from build123d import *

# Parameters (mm, degrees)
BOX016_W     = 28
BOX016_H     = 4
BOX016_DEPTH = 10
BOX004_W     = 30
BOX004_H     = 8
BOX004_DEPTH = 2.5
BOX003_W     = 30
BOX003_H     = 10
BOX003_DEPTH = 3.5
BOX002_W     = 30
BOX002_H     = 21
BOX002_DEPTH = 1


with BuildPart() as cubo016:
    # Box016 → Box016 (new body)
    with BuildSketch(Plane(origin=(-13, -14, 0), x_dir=(1, 0, 0), z_dir=(0, 0, 1))):
        with Locations((14, 2)):
            Rectangle(BOX016_W, BOX016_H)
    extrude(amount=BOX016_DEPTH)


with BuildPart() as cubo004:
    # Box004 → Box004 (new body)
    with BuildSketch(Plane(origin=(-14, -15, 0), x_dir=(1, 0, 0), z_dir=(0, 0, 1))):
        with Locations((15, 4)):
            Rectangle(BOX004_W, BOX004_H)
    extrude(amount=BOX004_DEPTH)


with BuildPart() as cubo003:
    # Box003 → Box003 (new body)
    with BuildSketch(Plane(origin=(-14, -16, 0), x_dir=(1, 0, 0), z_dir=(0, 0, 1))):
        with Locations((15, 5)):
            Rectangle(BOX003_W, BOX003_H)
    extrude(amount=BOX003_DEPTH)


with BuildPart() as cut008:
    # Box002 → Box002 (new body)
    with BuildSketch(Plane(origin=(-14, -21, 0), x_dir=(1, 0, 0), z_dir=(0, 0, 1))):
        with Locations((15, 10.5)):
            Rectangle(BOX002_W, BOX002_H)
    extrude(amount=BOX002_DEPTH)

    # Fusion001: union Cubo003
    add(cubo003.part)

    # Cut006: cut Cubo004
    add(cubo004.part, mode=Mode.SUBTRACT)

    # Cut008: cut Cubo016
    add(cubo016.part, mode=Mode.SUBTRACT)


solid = cut008.part
Verification items for the finished model (mm, model axes). A direction names the side the tool comes from. Give positions to 0.01 mm unless a question says otherwise; leave off trailing zeros. Loops run counter-clockwise (first coordinate to the right, second up) from the corner with the lowest first, then second, coordinate; pieces in that order, holes last.
1. Material ranges on probe 1 along Y at (x, z) = (14, 2.65); probe 2 along Y at (x, z) = (11.5, 1.65); probe 3 along Z at (x, y) = (-10, -2), recorded low to high.
Derived:
probe 1: y = -16 to -14, -10 to -6
probe 2: y = -16 to -15, -7 to -6
probe 3: z = 0 to 1
2. Cross-section at A-A on x = -0.5. Record the cut outline in (y, z).
Derived:
outline: (-21, 0) - (-15, 0) - (-15, 2.5) - (-14, 2.5) - (-14, 3.5) - (-16, 3.5) - (-16, 1) - (-21, 1) - close; (-10, 2.5) - (-7, 2.5) - (-7, 0) - (0, 0) - (0, 1) - (-6, 1) - (-6, 3.5) - (-10, 3.5) - close
3. Tool access check on faces 1 (the flat face through (1, -7, 1)), 2 (the flat face through (1, -16, 2)), 3 (the flat face through (1, -3, 0)), 4 (the flat face through (1, -14, 3)), 5 (the flat face through (1, -3, 1)). Record the directions out of +Z, -Z, +X, -X, +Y, -Y that give a thin tool (end or side, any length) a straight path to the whole face; none if there is none.
Derived:
face 1: -Z, +X, -X
face 2: +Z, +X, -X, -Y
face 3: -Z, +X, -X, +Y, -Y
face 4: +Z, -Z
face 5: +Z, +X, -X, +Y
4. Release check for a two-part mould opening along X. For faces 6 (the flat face through (1, -18, 1)), 7 (the flat face through (-13, -12, 3)), 8 (the flat face through (16, -11, 3)) record: +X half, -X half, draft (parallel to the pull), parting line (faces both ways), or undercut.
Derived:
face 6: draft
face 7: undercut
face 8: +X half
5. Cross-section at C-C on y = -5.25. Record the cut outline in (x, z), and give its area (3 significant figures).
Derived:
outline: (-14, 0) - (16, 0) - (16, 1) - (-14, 1) - close
area: 30.0 mm2
6. Go/stop test with flat-tipped pins: P1, Ø6.5, axis at x = 6, y = -2, coming from the +Z side; P2, Ø1, axis at x = -6.5, z = 2.5, coming from the +Y side; P3, Ø0.5, axis at x = -2, z = 3, coming from the -Y side. Record where each tip stops, or that it passes through.
Derived:
P1: stops at z = 1
P2: stops at y = -6
P3: stops at y = -16
7. Cross-section at B-B on z = 1.5. Record the cut outline in (x, y), and give its area (3 significant figures).
Derived:
outline: (-14, -16) - (16, -16) - (16, -15) - (-14, -15) - close; (-14, -7) - (16, -7) - (16, -6) - (-14, -6) - close
area: 60.0 mm2
